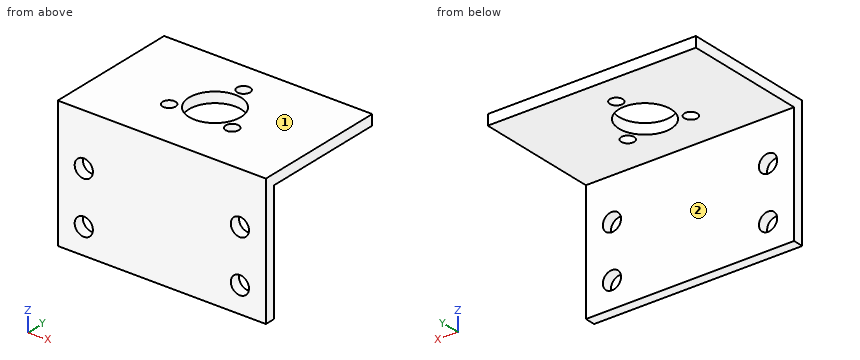
from build123d import *

# Parameters (mm, degrees)
SKETCH1_W           = 40
SKETCH1_H           = 25
BOSS_EXTRUDE1_DEPTH = 2
SKETCH2_W           = 40
SKETCH2_H           = 2
BOSS_EXTRUDE2_DEPTH = 24
SKETCH3_R           = 1.75
CUT_EXTRUDE1_DEPTH  = 36.103418637
LPATTERN1_COUNT     = 2
LPATTERN1_PITCH     = 10
SKETCH5_R           = 5
CUT_EXTRUDE2_DEPTH  = 42.243181255
SKETCH6_R           = 1.25
CUT_EXTRUDE3_DEPTH  = 42.243181255
CIRPATTERN1_COUNT   = 3


with BuildPart() as part:
    # Sketch1 → Boss-Extrude1 (new body)
    with BuildSketch(Plane(origin=(0, 0, 0), x_dir=(1, 0, 0), z_dir=(0, 1, 0))):
        Rectangle(SKETCH1_W, SKETCH1_H)
    extrude(amount=BOSS_EXTRUDE1_DEPTH)

    # Sketch2 → Boss-Extrude2 (add)
    with BuildSketch(Plane(origin=(0, 2, 0), x_dir=(1, 0, 0), z_dir=(0, 1, 0))):
        with Locations((0, -11.5)):
            Rectangle(SKETCH2_W, SKETCH2_H)
    extrude(amount=BOSS_EXTRUDE2_DEPTH)

    # Sketch3 → Cut-Extrude1 (cut, through all)
    with BuildSketch(Plane.XZ):
        with Locations(Location((-15, -7.5, 0), (0, 0, 270))):
            Circle(SKETCH3_R)
        with Locations(Location((15, -7.5, 0), (0, 0, 270))):
            Circle(SKETCH3_R)
    cut_extrude1 = extrude(amount=-CUT_EXTRUDE1_DEPTH, mode=Mode.SUBTRACT)

    # LPattern1: Cut-Extrude1 ×2
    with Locations(*[(0, 0, i * LPATTERN1_PITCH) for i in range(1, LPATTERN1_COUNT)]):
        add(cut_extrude1, mode=Mode.SUBTRACT)

    # Sketch5 → Cut-Extrude2 (cut, through all)
    with BuildSketch(Plane.XY.offset(12.5)):
        with Locations((0, 13)):
            Circle(SKETCH5_R)
    extrude(amount=-CUT_EXTRUDE2_DEPTH, mode=Mode.SUBTRACT)

    # Sketch6 → Cut-Extrude3 (cut, through all)
    with BuildSketch(Plane.XY.offset(12.5)):
        with Locations((0, 20)):
            Circle(SKETCH6_R)
    cut_extrude3 = extrude(amount=-CUT_EXTRUDE3_DEPTH, mode=Mode.SUBTRACT)

    # CirPattern1: Cut-Extrude3 ×3 about axis
    cirpattern1_axis = Axis((0, 13, 0), (0, 0, 1))
    for i in range(1, CIRPATTERN1_COUNT):
        add(cut_extrude3.rotate(cirpattern1_axis, i * 360 / CIRPATTERN1_COUNT), mode=Mode.SUBTRACT)


solid = part.part
Design review of the part built by this model. Coordinates are the model's own, in mm. Face numbers are marked on the shaded views. A direction names the side the tool comes from. Coordinates: 2 decimals unless noted, no trailing zeros. Order: outer loops, then holes, each group sorted by start corner. A loop starts at its lowest first (then second) coordinate and runs counter-clockwise, first axis right, second up. Notation, with made-up numbers: M 89,84 L 122,84 A21 cw 122,106 Z; hole C 43,61.5 d5. An arc over 180 degrees is marked long. Use a Markdown table: item, result.
(1) For P1, Ø4, axis at x = 6.06, y = 9.5, coming from the -Z side; P2, Ø6, axis at x = -3, z = -6, coming from the +Y side, all flat-tipped, find the tip position at first contact; note any pin that passes through.
Worked answers:
| item | result |
|---|---|
| P1 | stops at z = 10.5 |
| P2 | stops at y = 2 |
(2) Add section C-C (z = 2.5). Give the boundary of the cut face in (x, y), then the cut area to 3 significant figures.
Worked answers:
| item | result |
|---|---|
| outline | M -20,0 L -16.75,0 L -16.75,2 L -20,2 Z; M -13.25,0 L 13.25,0 L 13.25,2 L -13.25,2 Z; M 16.75,0 L 20,0 L 20,2 L 16.75,2 Z |
| area | 66.0 mm2 |
(3) For the marked faces 1 and 2, list the 3-axis set-ups (+Z, -Z, +X, -X, +Y, -Y) from which the entire face can be reached by the end or side of a thin tool; tool diameter is ignored.
Worked answers:
| item | result |
|---|---|
| face 1 | +Z, +X, -X, +Y, -Y |
| face 2 | -Z, +X, -X, +Y |
(4) Add section A-A (y = 16). Give the boundary of the cut face in (x, z), then the cut area to 3 significant figures.
Worked answers:
| item | result |
|---|---|
| outline | M -20,10.5 L -4,10.5 L -4,12.5 L -20,12.5 Z; M 4,10.5 L 20,10.5 L 20,12.5 L 4,12.5 Z |
| area | 64.0 mm2 |
(5) Add section D-D (y = 9.5). Give the boundary of the cut face in (x, z), then the cut area to 3 significant figures.
Worked answers:
| item | result |
|---|---|
| outline | M -20,10.5 L -7.31,10.5 L -7.31,12.5 L -20,12.5 Z; M -4.81,10.5 L -3.57,10.5 L -3.57,12.5 L -4.81,12.5 Z; M 3.57,10.5 L 4.81,10.5 L 4.81,12.5 L 3.57,12.5 Z; M 7.31,10.5 L 20,10.5 L 20,12.5 L 7.31,12.5 Z |
| area | 55.7 mm2 |
(6) Wall thickness on probe 1 along X at (y, z) = (1.15, 2.5); probe 2 along Y at (x, z) = (0, 11.1); probe 3 along X at (y, z) = (9.5, 11.45): over which ranges is each line inside the solid? List them lowest first.
Worked answers:
| item | result |
|---|---|
| probe 1 | x = -20 to -16.75, -13.25 to 13.25, 16.75 to 20 |
| probe 2 | y = 0 to 8, 18 to 18.75, 21.25 to 26 |
| probe 3 | x = -20 to -7.31, -4.81 to -3.57, 3.57 to 4.81, 7.31 to 20 |
(7) Add section B-B (x = -15). Give the boundary of the cut face in (y, z), then the cut area to 3 significant figures.
Worked answers:
| item | result |
|---|---|
| outline | M 0,-12.5 L 2,-12.5 L 2,-9.25 L 0,-9.25 Z; M 0,-5.75 L 2,-5.75 L 2,0.75 L 0,0.75 Z; M 0,4.25 L 2,4.25 L 2,10.5 L 26,10.5 L 26,12.5 L 0,12.5 Z |
| area | 84.0 mm2 |
